Check sheet for the modelled part. Datum: model origin and axes. Units: mm. A direction names the side the tool comes from. Give positions to 0.01 mm unless a question says otherwise; leave off trailing zeros. Order: outer loops, then holes, each group sorted by start corner. A loop starts at its lowest first (then second) coordinate and runs counter-clockwise, first axis right, second up.
Item 1: Sectioned sample at C-C on z = 8.5. Record the boundary of the cut face in (x, y), and give its area (3 significant figures).
Item 2: Access from +Z, -Z, +X, -X, +Y, -Y to the whole of each face (thin tool, end or side, straight path). Record for faces 1 (the flat face through (-16.43, 2, -14.07)), 2 (the flat face through (-0.2, -11.2, 19.5)), 3 (the cylindrical face through (15.32, -4.59, -16.75)).
Item 3: Sectioned sample at D-D on x = 14.5. Count the separate pieces of the cut face and the enclosed holes in it, and give its area (3 significant figures).
Item 4: Release check for a two-part mould opening along Z. For faces 4 (the flat face through (0, -5, 25)), 5 (the flat face through (-20, -16, 0)), 6 (the cylindrical face through (-23.859, -5.353, -23.797)), 7 (the flat face through (11.23, -7, -3.11)) record: released by +Z, released by -Z, zero draft, split by the parting line, or undercut.
Item 5: Material ranges on line 1 along X through (y, z) = (-2.5, 0); line 2 along X through (y, z) = (3.95, 15.25); line 3 along Z through (x, y) = (12.5, -5), recorded low to high.
Item 6: Sectioned sample at B-B on x = 6.5. Record the boundary of the cut face in (y, z).
Item 7: Sectioned sample at A-A on y = -10. Record the boundary of the cut face in (x, z), and give its area (3 significant figures).
Item 8: Gauge pin test, flat ends, axial feed: P1, Ø4, axis at x = -15.25, z = -15.25, coming from the +Y side; P2, Ø6.5, axis at x = -15.25, z = 15.25, coming from the -Y side; P3, Ø2, axis at y = 24.5, z = -0.5, coming from the +X side (3 decimals). Record the tip position at first contact, or that the pin passes through.
from build123d import *

# Parameters (mm, degrees)
BOSS_EXTRUDE1_DEPTH     = 16
SKETCH4_3_R             = 2.75
SKETCH4_3_R_2           = 1.5
BOSS_EXTRUDE2_DEPTH     = 11
SKETCH4_4_R             = 13.7
BOSS_EXTRUDE3_DEPTH     = 7
BOSS_EXTRUDE4_START     = 5
BOSS_EXTRUDE4_DEPTH     = 5
BOSS_EXTRUDE5_START     = 5
SKETCH4_6_R             = 15.875
BOSS_EXTRUDE5_DEPTH     = 30
CUT_EXTRUDE1_DEPTH      = 50.749371855
CUT_EXTRUDE1_DEPTH_BACK = 7
SKETCH4_7_R             = 11.5
CUT_EXTRUDE4_DEPTH      = 50.749371855
CUT_EXTRUDE4_DEPTH_BACK = 50.749371855
SKETCH4_8_R             = 1.5
CUT_EXTRUDE5_START      = 5
SKETCH4_9_R             = 2.75
CUT_EXTRUDE5_DEPTH      = 3
SKETCH4_10_W            = 17
SKETCH4_10_H            = 5.5
BOSS_EXTRUDE6_DEPTH     = 12.5
FILLET1_R               = 1


with BuildPart() as part:
    # Sketch4 → Boss-Extrude1 (new body)
    with BuildSketch(Plane(origin=(0, 0, 0), x_dir=(1, 0, 0), z_dir=(0, 1, 0))):
        with BuildLine():
            Line((8.5, -25), (21, -25))
            ThreePointArc((21, -25), (23.828427125, -23.828427125), (25, -21))
            Line((25, -21), (25, 21))
            ThreePointArc((25, 21), (23.828427125, 23.828427125), (21, 25))
            Line((21, 25), (-21, 25))
            ThreePointArc((-21, 25), (-23.828427125, 23.828427125), (-25, 21))
            Line((-25, 21), (-25, -21))
            ThreePointArc((-25, -21), (-23.828427125, -23.828427125), (-21, -25))
            Line((-21, -25), (-8.5, -25))
            Line((-8.5, -25), (-8.5, -19.5))
            Line((-8.5, -19.5), (-15.5, -19.5))
            ThreePointArc((-15.5, -19.5), (-18.328427125, -18.328427125), (-19.5, -15.5))
            Line((-19.5, -15.5), (-19.5, 15.5))
            ThreePointArc((-19.5, 15.5), (-18.328427125, 18.328427125), (-15.5, 19.5))
            Line((-15.5, 19.5), (-5.5, 19.5))
            Line((-5.5, 19.5), (-5.5, 22))
            Line((-5.5, 22), (5.5, 22))
            Line((5.5, 22), (5.5, 19.5))
            Line((5.5, 19.5), (15.5, 19.5))
            ThreePointArc((15.5, 19.5), (18.328427125, 18.328427125), (19.5, 15.5))
            Line((19.5, 15.5), (19.5, -15.5))
            ThreePointArc((19.5, -15.5), (18.328427125, -18.328427125), (15.5, -19.5))
            Line((15.5, -19.5), (8.5, -19.5))
            Line((8.5, -19.5), (8.5, -25))
        make_face()
    extrude(amount=-BOSS_EXTRUDE1_DEPTH)

    # Sketch4<3> → Boss-Extrude2 (add)
    # profile 1 of 7: a face of its own
    with BuildSketch(Plane(origin=(0, 0, 0), x_dir=(1, 0, 0), z_dir=(0, 1, 0))):
        with BuildLine():
            Line((-8.5, -19.5), (8.5, -19.5))
            Line((8.5, -19.5), (15.5, -19.5))
            ThreePointArc((15.5, -19.5), (18.328427125, -18.328427125), (19.5, -15.5))
            Line((19.5, -15.5), (19.5, 15.5))
            ThreePointArc((19.5, 15.5), (18.328427125, 18.328427125), (15.5, 19.5))
            Line((15.5, 19.5), (5.5, 19.5))
            Line((5.5, 19.5), (5.5, 17.139136501))
            ThreePointArc((5.5, 17.139136501), (14.543039572, 10.606601718), (18, 0))
            ThreePointArc((18, 0), (-10.606601718, -14.543039572), (-5.5, 17.139136501))
            Line((-5.5, 17.139136501), (-5.5, 19.5))
            Line((-5.5, 19.5), (-15.5, 19.5))
            ThreePointArc((-15.5, 19.5), (-18.328427125, 18.328427125), (-19.5, 15.5))
            Line((-19.5, 15.5), (-19.5, -15.5))
            ThreePointArc((-19.5, -15.5), (-18.328427125, -18.328427125), (-15.5, -19.5))
            Line((-15.5, -19.5), (-8.5, -19.5))
        make_face()
        with Locations((-15.25, -15.25)):
            Circle(SKETCH4_3_R, mode=Mode.SUBTRACT)
        with Locations((15.25, -15.25)):
            Circle(SKETCH4_3_R, mode=Mode.SUBTRACT)
        with Locations((-15.25, 15.25)):
            Circle(SKETCH4_3_R, mode=Mode.SUBTRACT)
        with Locations((15.25, 15.25)):
            Circle(SKETCH4_3_R, mode=Mode.SUBTRACT)
    # profile 2 of 7: a face of its own
    with BuildSketch(Plane(origin=(0, 0, 0), x_dir=(1, 0, 0), z_dir=(0, 1, 0))):
        with BuildLine():
            Line((-8.5, -19.5), (8.5, -19.5))
            Line((8.5, -19.5), (15.5, -19.5))
            ThreePointArc((15.5, -19.5), (18.328427125, -18.328427125), (19.5, -15.5))
            Line((19.5, -15.5), (19.5, 15.5))
            ThreePointArc((19.5, 15.5), (18.328427125, 18.328427125), (15.5, 19.5))
            Line((15.5, 19.5), (5.5, 19.5))
            Line((5.5, 19.5), (5.5, 17.139136501))
            ThreePointArc((5.5, 17.139136501), (14.543039572, 10.606601718), (18, 0))
            ThreePointArc((18, 0), (-10.606601718, -14.543039572), (-5.5, 17.139136501))
            Line((-5.5, 17.139136501), (-5.5, 19.5))
            Line((-5.5, 19.5), (-15.5, 19.5))
            ThreePointArc((-15.5, 19.5), (-18.328427125, 18.328427125), (-19.5, 15.5))
            Line((-19.5, 15.5), (-19.5, -15.5))
            ThreePointArc((-19.5, -15.5), (-18.328427125, -18.328427125), (-15.5, -19.5))
            Line((-15.5, -19.5), (-8.5, -19.5))
        make_face()
        with Locations((-15.25, -15.25)):
            Circle(SKETCH4_3_R, mode=Mode.SUBTRACT)
        with Locations((15.25, -15.25)):
            Circle(SKETCH4_3_R, mode=Mode.SUBTRACT)
        with Locations((-15.25, 15.25)):
            Circle(SKETCH4_3_R, mode=Mode.SUBTRACT)
        with Locations((15.25, 15.25)):
            Circle(SKETCH4_3_R, mode=Mode.SUBTRACT)
    # profile 3 of 7: a face of its own
    with BuildSketch(Plane(origin=(0, 0, 0), x_dir=(1, 0, 0), z_dir=(0, 1, 0))):
        with BuildLine():
            Line((-8.5, -19.5), (8.5, -19.5))
            Line((8.5, -19.5), (15.5, -19.5))
            ThreePointArc((15.5, -19.5), (18.328427125, -18.328427125), (19.5, -15.5))
            Line((19.5, -15.5), (19.5, 15.5))
            ThreePointArc((19.5, 15.5), (18.328427125, 18.328427125), (15.5, 19.5))
            Line((15.5, 19.5), (5.5, 19.5))
            Line((5.5, 19.5), (5.5, 17.139136501))
            ThreePointArc((5.5, 17.139136501), (14.543039572, 10.606601718), (18, 0))
            ThreePointArc((18, 0), (-10.606601718, -14.543039572), (-5.5, 17.139136501))
            Line((-5.5, 17.139136501), (-5.5, 19.5))
            Line((-5.5, 19.5), (-15.5, 19.5))
            ThreePointArc((-15.5, 19.5), (-18.328427125, 18.328427125), (-19.5, 15.5))
            Line((-19.5, 15.5), (-19.5, -15.5))
            ThreePointArc((-19.5, -15.5), (-18.328427125, -18.328427125), (-15.5, -19.5))
            Line((-15.5, -19.5), (-8.5, -19.5))
        make_face()
        with Locations((-15.25, -15.25)):
            Circle(SKETCH4_3_R, mode=Mode.SUBTRACT)
        with Locations((15.25, -15.25)):
            Circle(SKETCH4_3_R, mode=Mode.SUBTRACT)
        with Locations((-15.25, 15.25)):
            Circle(SKETCH4_3_R, mode=Mode.SUBTRACT)
        with Locations((15.25, 15.25)):
            Circle(SKETCH4_3_R, mode=Mode.SUBTRACT)
    # profile 4 of 7: a face of its own
    with BuildSketch(Plane(origin=(0, 0, 0), x_dir=(1, 0, 0), z_dir=(0, 1, 0))):
        with Locations((-15.25, -15.25)):
            Circle(SKETCH4_3_R)
        with Locations(Location((-15.25, -15.25, 0), (0, 0, 270))):
            Circle(SKETCH4_3_R_2, mode=Mode.SUBTRACT)
    # profile 5 of 7: a face of its own
    with BuildSketch(Plane(origin=(0, 0, 0), x_dir=(1, 0, 0), z_dir=(0, 1, 0))):
        with Locations((15.25, -15.25)):
            Circle(SKETCH4_3_R)
        with Locations(Location((15.25, -15.25, 0), (0, 0, 270))):
            Circle(SKETCH4_3_R_2, mode=Mode.SUBTRACT)
    # profile 6 of 7: a face of its own
    with BuildSketch(Plane(origin=(0, 0, 0), x_dir=(1, 0, 0), z_dir=(0, 1, 0))):
        with Locations((15.25, 15.25)):
            Circle(SKETCH4_3_R)
        with Locations(Location((15.25, 15.25, 0), (0, 0, 270))):
            Circle(SKETCH4_3_R_2, mode=Mode.SUBTRACT)
    # profile 7 of 7: a face of its own
    with BuildSketch(Plane(origin=(0, 0, 0), x_dir=(1, 0, 0), z_dir=(0, 1, 0))):
        with Locations((-15.25, 15.25)):
            Circle(SKETCH4_3_R)
        with Locations(Location((-15.25, 15.25, 0), (0, 0, 270))):
            Circle(SKETCH4_3_R_2, mode=Mode.SUBTRACT)
    extrude(amount=-BOSS_EXTRUDE2_DEPTH)



with BuildPart() as body_2:
    # Sketch4<4> → Boss-Extrude3 (new body)
    with BuildSketch(Plane(origin=(0, 0, 0), x_dir=(1, 0, 0), z_dir=(0, 1, 0))):
        with Locations(Location((0, 0, 0), (0, 0, 270))):
            Circle(SKETCH4_4_R)
    extrude(amount=-BOSS_EXTRUDE3_DEPTH)

    # Sketch4<5> → Boss-Extrude4 (add)
    with BuildSketch(Plane(origin=(0, 0, 0), x_dir=(1, 0, 0), z_dir=(0, 1, 0)).offset(BOSS_EXTRUDE4_START)):
        with BuildLine():
            Line((21, -25), (-21, -25))
            ThreePointArc((-21, -25), (-23.828427125, -23.828427125), (-25, -21))
            Line((-25, -21), (-25, 21))
            ThreePointArc((-25, 21), (-23.828427125, 23.828427125), (-21, 25))
            Line((-21, 25), (21, 25))
            ThreePointArc((21, 25), (23.828427125, 23.828427125), (25, 21))
            Line((25, 21), (25, -21))
            ThreePointArc((25, -21), (23.828427125, -23.828427125), (21, -25))
        make_face()
    extrude(amount=-BOSS_EXTRUDE4_DEPTH)

    # Sketch4<6> → Boss-Extrude5 (add)
    with BuildSketch(Plane(origin=(0, 0, 0), x_dir=(1, 0, 0), z_dir=(0, 1, 0)).offset(BOSS_EXTRUDE5_START)):
        with Locations(Location((0, 0, 0), (0, 0, 270))):
            Circle(SKETCH4_6_R)
    extrude(amount=BOSS_EXTRUDE5_DEPTH)

    # Sketch4<7> → Cut-Extrude1 (cut, two sides: drawn at the far end of the back side and taken through both)
    with BuildSketch(Plane(origin=(0, 0, 0), x_dir=(1, 0, 0), z_dir=(0, 1, 0)).offset(-CUT_EXTRUDE1_DEPTH_BACK)):
        with Locations(Location((0, 0, 0), (0, 0, 270))):
            Circle(SKETCH4_7_R)
    extrude(amount=CUT_EXTRUDE1_DEPTH + CUT_EXTRUDE1_DEPTH_BACK, mode=Mode.SUBTRACT)

    # Sketch4<8> → Cut-Extrude4 (cut, two sides: drawn at the far end of the back side and taken through both)
    with BuildSketch(Plane(origin=(0, 0, 0), x_dir=(1, 0, 0), z_dir=(0, 1, 0)).offset(-CUT_EXTRUDE4_DEPTH_BACK)):
        with Locations(Location((15.25, -15.25, 0), (0, 0, 270))):
            Circle(SKETCH4_8_R)
        with Locations(Location((-15.25, -15.25, 0), (0, 0, 270))):
            Circle(SKETCH4_8_R)
        with Locations(Location((-15.25, 15.25, 0), (0, 0, 270))):
            Circle(SKETCH4_8_R)
        with Locations(Location((15.25, 15.25, 0), (0, 0, 270))):
            Circle(SKETCH4_8_R)
    extrude(amount=CUT_EXTRUDE4_DEPTH + CUT_EXTRUDE4_DEPTH_BACK, mode=Mode.SUBTRACT)

    # Sketch4<9> → Cut-Extrude5 (cut)
    with BuildSketch(Plane(origin=(0, 0, 0), x_dir=(1, 0, 0), z_dir=(0, 1, 0)).offset(CUT_EXTRUDE5_START)):
        with Locations(Location((-15.25, -15.25, 0), (0, 0, 270))):
            Circle(SKETCH4_9_R)
        with Locations(Location((15.25, -15.25, 0), (0, 0, 270))):
            Circle(SKETCH4_9_R)
        with Locations(Location((15.25, 15.25, 0), (0, 0, 270))):
            Circle(SKETCH4_9_R)
        with Locations(Location((-15.25, 15.25, 0), (0, 0, 270))):
            Circle(SKETCH4_9_R)
    extrude(amount=-CUT_EXTRUDE5_DEPTH, mode=Mode.SUBTRACT)


with BuildPart() as part_1:
    add(part.part)

    add(body_2.part)  # Boss-Extrude6 merges body 2
    # Sketch4<10> → Boss-Extrude6 (add)
    with BuildSketch(Plane(origin=(0, 0, 0), x_dir=(1, 0, 0), z_dir=(0, 1, 0))):
        with Locations((0, -22.25)):
            Rectangle(SKETCH4_10_W, SKETCH4_10_H)
    extrude(amount=-BOSS_EXTRUDE6_DEPTH)

    # Fillet1
    fillet1_edges = [part_1.edges().sort_by_distance(p)[0] for p in [
        (0, -12.5, 19.5),
        (0, -12.5, 25),
        (-8.5, -14.25, 19.5),
        (-8.5, -14.25, 25),
        (8.5, -14.25, 25),
        (8.5, -14.25, 19.5),
    ]]
    fillet(fillet1_edges, radius=FILLET1_R)


solid = part_1.part
Report:
1. outline: (-25, -16) - (-19.5, -16) - (-19.5, -11) - (-15.87, -11) - (-15.87, 0) - (-10.74, 0) - (-10.74, -7) - (-7.75, -7) - (-7.75, 35) - (-13.41, 35) - (-13.41, 5) - (-25, 5) - close; (7.75, -7) - (10.74, -7) - (10.74, 0) - (15.87, 0) - (15.87, -11) - (19.5, -11) - (19.5, -16) - (25, -16) - (25, 5) - (13.41, 5) - (13.41, 35) - (7.75, 35) - close
1. area: 810 mm2
2. face 1: +Y
2. face 2: -Y
2. face 3: +Y, -Y
3. separate pieces: 3
3. enclosed holes: 0
3. area: 909 mm2
4. face 4: released by +Z
4. face 5: zero draft
4. face 6: released by -Z
4. face 7: undercut
5. line 1: x = -25 to -18, -13.7 to -11.5, 11.5 to 13.7, 18 to 25
5. line 2: x = -25 to -18, -12.5 to 12.5, 18 to 25
5. line 3: z = -25 to -12.95, -5.61 to 5.61, 12.95 to 25
6. outline: (-16, -25) - (5, -25) - (5, -14.48) - (35, -14.48) - (35, -9.49) - (-7, -9.49) - (-7, -12.06) - (0, -12.06) - (0, -16.79) - (-11, -16.79) - (-11, -19.5) - (-16, -19.5) - close; (-12.5, 20.5) arc R1 ccw to (-11.5, 19.5) - (-11, 19.5) - (-11, 16.79) - (0, 16.79) - (0, 12.06) - (-7, 12.06) - (-7, 9.49) - (35, 9.49) - (35, 14.48) - (5, 14.48) - (5, 25) - (-11.5, 25) arc R1 ccw to (-12.5, 24) - close
7. outline: (-25, -21) arc R4 ccw to (-21, -25) - (21, -25) arc R4 ccw to (25, -21) - (25, 21) arc R4 ccw to (21, 25) - (-21, 25) arc R4 ccw to (-25, 21) - close; hole circle Ø3 at (-15.25, -15.25); hole circle Ø3 at (-15.25, 15.25); hole (-5.5, -22) - (5.5, -22) - (5.5, -17.14) arc R18 ccw (long way) to (-5.5, -17.14) - close; hole circle Ø3 at (15.25, -15.25); hole circle Ø3 at (15.25, 15.25)
7. area: 1,390 mm2
8. P1: stops at y = 2
8. P2: stops at y = -11
8. P3: stops at x = 15.875
